from build123d import *

# Parameters (mm, degrees)
SKETCH1_R           = 12.37
BOSS_EXTRUDE1_DEPTH = 10
SKETCH2_R           = 19.423188446
BOSS_EXTRUDE2_DEPTH = 50
SKETCH4_R           = 12.37
BOSS_EXTRUDE3_DEPTH = 10
BOSS_EXTRUDE4_START = -5
SKETCH5_W           = 7.115833501
SKETCH5_H           = 0.529627629
BOSS_EXTRUDE4_DEPTH = 40
CIRPATTERN1_COUNT   = 15
SKETCH6_R           = 9.521283716
CUT_EXTRUDE1_DEPTH  = 5
CUT_EXTRUDE2_START  = -5
SKETCH7_R           = 9.521283716
CUT_EXTRUDE2_DEPTH  = 5
SKETCH8_R           = 7.481646465
BOSS_EXTRUDE5_DEPTH = 7
BOSS_EXTRUDE6_START = 7
SKETCH9_R           = 7.481646465
BOSS_EXTRUDE6_DEPTH = 7


with BuildPart() as part:
    # Sketch1 → Boss-Extrude1 (new body)
    with BuildSketch(Plane.XY):
        Circle(SKETCH1_R)
    extrude(amount=BOSS_EXTRUDE1_DEPTH)

    # Sketch2 → Boss-Extrude2 (add)
    with BuildSketch(Plane.XY.offset(10)):
        Circle(SKETCH2_R)
    extrude(amount=BOSS_EXTRUDE2_DEPTH)

    # Sketch4 → Boss-Extrude3 (add)
    with BuildSketch(Plane.XY.offset(60)):
        Circle(SKETCH4_R)
    extrude(amount=BOSS_EXTRUDE3_DEPTH)

    # Sketch5 → Boss-Extrude4 (add)
    with BuildSketch(Plane.XY.offset(60).offset(BOSS_EXTRUDE4_START)):
        with Locations((-0.343381899, 19.42015289)):
            Rectangle(SKETCH5_W, SKETCH5_H)
    boss_extrude4 = extrude(amount=-BOSS_EXTRUDE4_DEPTH)

    # CirPattern1: Boss-Extrude4 ×15 about axis
    cirpattern1_axis = Axis((0, 0, 0), (0, 0, -1))
    for i in range(1, CIRPATTERN1_COUNT):
        add(boss_extrude4.rotate(cirpattern1_axis, i * 360 / CIRPATTERN1_COUNT))

    # Sketch6 → Cut-Extrude1 (cut)
    with BuildSketch(Plane.XY.offset(70)):
        Circle(SKETCH6_R)
    extrude(amount=-CUT_EXTRUDE1_DEPTH, mode=Mode.SUBTRACT)

    # Sketch7 → Cut-Extrude2 (cut)
    with BuildSketch(Plane(origin=(0, 0, 0), x_dir=(-1, 0, 0), z_dir=(0, 0, -1)).offset(CUT_EXTRUDE2_START)):
        with Locations(Location((0, 0, 0), (0, 0, 180))):
            Circle(SKETCH7_R)
    extrude(amount=CUT_EXTRUDE2_DEPTH, mode=Mode.SUBTRACT)

    # Sketch8 → Boss-Extrude5 (add)
    with BuildSketch(Plane(origin=(0, 0, 5), x_dir=(-1, 0, 0), z_dir=(0, 0, -1))):
        Circle(SKETCH8_R)
    extrude(amount=BOSS_EXTRUDE5_DEPTH)

    # Sketch9 → Boss-Extrude6 (add)
    with BuildSketch(Plane.XY.offset(65).offset(BOSS_EXTRUDE6_START)):
        with Locations(Location((0, 0, 0), (0, 0, 180))):
            Circle(SKETCH9_R)
    extrude(amount=-BOSS_EXTRUDE6_DEPTH)


solid = part.part
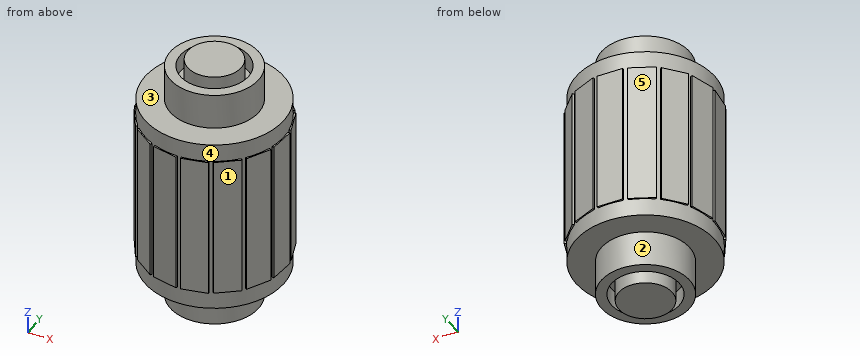
Model file for the job. Use its own axes, mm. Face numbers are marked on the shaded views. A direction names the side the tool comes from. Give positions to 0.01 mm unless a question says otherwise; leave off trailing zeros. Write each loop counter-clockwise with the first axis right and the second up, starting at its lowest first coordinate (ties: lowest second). Pieces come first, ordered by that corner, then holes. Notation, with made-up numbers: M 55.25,-11 L 60.25,-11 A17 ccw 60.25,17 Z; hole C 84.25,-23 d9. An arc over 180 degrees is marked long. One line per item, written item: value. Start each with the question number.
Q1. Drop flat-ended pins along their axis: pin 1 Ø2 at (y, z) = (-4, 41.5) entering from -X; pin 2 Ø1.7 at (x, y) = (8, 18) entering from -Z; pin 3 Ø12 at (y, z) = (-15, 7) entering from -X. Give the stop position or say it passes through.
Q2. 3-axis set-ups, long thin cutter, end or side, ignore diameter. For the marked faces 1, 2, 3, 4 and 5: which of +Z, -Z, +X, -X, +Y, -Y reach the whole face in a straight line?
Q3. Saw through at A-A, the plane y = -11. Write the cut outline in (x, z).
Q4. Probe probe 1 along Y at (x, z) = (0, 3); probe 2 along Z at (x, y) = (13, 7.5); probe 3 along Z at (x, y) = (10, -5.5). List the from-to ranges inside material, lowest first. Write a range as [from, to].
Output values:
1. pin 1: stops at x = -19.48
1. pin 2: stops at z = 10
1. pin 3: stops at x = -16.77
2. face 1: +Z, -Z, +X, -Y
2. face 2: -Z
2. face 3: +Z
2. face 4: none
2. face 5: +Z, -Z, -X, +Y
3. outline: M -16.38,15 L -16.01,15 L -16.01,10 L -5.66,10 L -5.66,0 L 5.66,0 L 5.66,10 L 16.01,10 L 16.01,15 L 16.38,15 L 16.38,55 L 16.01,55 L 16.01,60 L 5.66,60 L 5.66,70 L -5.66,70 L -5.66,60 L -16.01,60 L -16.01,55 L -16.38,55 Z
4. probe 1: y = [-12.37, -9.52], [-7.48, 7.48], [9.52, 12.37]
4. probe 2: z = [10, 60]
4. probe 3: z = [0, 70]
